```python
from build123d import *

# Parameters (mm, degrees)
SKETCH2_R           = 1.5
BOSS_EXTRUDE1_DEPTH = 2
SKETCH2_4_R         = 4
SKETCH2_4_R_2       = 1.5
BOSS_EXTRUDE2_DEPTH = 20
CUT_EXTRUDE1_START  = 20
SKETCH2_5_R         = 4
SKETCH2_5_R_2       = 3
CUT_EXTRUDE1_DEPTH  = 5


with BuildPart() as part:
    # Sketch2 → Boss-Extrude1 (new body)
    with BuildSketch(Plane(origin=(0, 0, 0), x_dir=(1, 0, 0), z_dir=(0, 1, 0))):
        with BuildLine():
            ThreePointArc((22, -5.5), (27.5, 0), (22, 5.5))
            ThreePointArc((22, 5.5), (16.628166969, 6.705737819), (12.286949473, 10.091623885))
            ThreePointArc((12.286949473, 10.091623885), (11.242997821, 11.242997821), (10.091623885, 12.286949473))
            ThreePointArc((10.091623885, 12.286949473), (6.705737819, 16.628166969), (5.5, 22))
            ThreePointArc((5.5, 22), (0, 27.5), (-5.5, 22))
            ThreePointArc((-5.5, 22), (-6.705737819, 16.628166969), (-10.091623885, 12.286949473))
            ThreePointArc((-10.091623885, 12.286949473), (-11.242997821, 11.242997821), (-12.286949473, 10.091623885))
            ThreePointArc((-12.286949473, 10.091623885), (-16.628166969, 6.705737819), (-22, 5.5))
            ThreePointArc((-22, 5.5), (-27.5, 0), (-22, -5.5))
            ThreePointArc((-22, -5.5), (-16.628166969, -6.705737819), (-12.286949473, -10.091623885))
            ThreePointArc((-12.286949473, -10.091623885), (-11.242997821, -11.242997821), (-10.091623885, -12.286949473))
            ThreePointArc((-10.091623885, -12.286949473), (-6.705737819, -16.628166969), (-5.5, -22))
            ThreePointArc((-5.5, -22), (0, -27.5), (5.5, -22))
            ThreePointArc((5.5, -22), (6.705737819, -16.628166969), (10.091623885, -12.286949473))
            ThreePointArc((10.091623885, -12.286949473), (11.242997821, -11.242997821), (12.286949473, -10.091623885))
            ThreePointArc((12.286949473, -10.091623885), (16.628166969, -6.705737819), (22, -5.5))
        make_face()
        with Locations(Location((-22, 0, 0), (0, 0, 270))):
            Circle(SKETCH2_R, mode=Mode.SUBTRACT)
        with Locations(Location((-9.192388155, -9.192388155, 0), (0, 0, 270))):
            Circle(SKETCH2_R, mode=Mode.SUBTRACT)
        with BuildLine():
            Line((7.526291329, 6.431558041), (7.526291329, 0))
            Line((7.526291329, 0), (7.526291329, -6.388653952))
            Line((7.526291329, -6.388653952), (7.562744256, -6.388653952))
            ThreePointArc((7.562744256, -6.388653952), (-1e-09, -9.9), (-7.562744258, -6.38865395))
            Line((-7.562744258, -6.38865395), (-7.526291329, -6.388653952))
            Line((-7.526291329, -6.388653952), (-7.526291329, 6.431558041))
            ThreePointArc((-7.526291329, 6.431558041), (0, 9.9), (7.526291329, 6.431558041))
        make_face(mode=Mode.SUBTRACT)
        with Locations(Location((0, -22, 0), (0, 0, 270))):
            Circle(SKETCH2_R, mode=Mode.SUBTRACT)
        with Locations(Location((9.192388155, -9.192388155, 0), (0, 0, 270))):
            Circle(SKETCH2_R, mode=Mode.SUBTRACT)
        with Locations(Location((22, 0, 0), (0, 0, 270))):
            Circle(SKETCH2_R, mode=Mode.SUBTRACT)
        with Locations(Location((-9.192388155, 9.192388155, 0), (0, 0, 270))):
            Circle(SKETCH2_R, mode=Mode.SUBTRACT)
        with Locations(Location((9.192388155, 9.192388155, 0), (0, 0, 270))):
            Circle(SKETCH2_R, mode=Mode.SUBTRACT)
        with Locations(Location((0, 22, 0), (0, 0, 270))):
            Circle(SKETCH2_R, mode=Mode.SUBTRACT)
    extrude(amount=BOSS_EXTRUDE1_DEPTH)

    # Sketch2<4> → Boss-Extrude2 (add)
    with BuildSketch(Plane(origin=(0, 0, 0), x_dir=(1, 0, 0), z_dir=(0, 1, 0))):
        with Locations(Location((22, 0, 0), (0, 0, 270))):
            Circle(SKETCH2_4_R)
        with Locations(Location((22, 0, 0), (0, 0, 270))):
            Circle(SKETCH2_4_R_2, mode=Mode.SUBTRACT)
        with Locations(Location((0, -22, 0), (0, 0, 270))):
            Circle(SKETCH2_4_R)
        with Locations(Location((0, -22, 0), (0, 0, 270))):
            Circle(SKETCH2_4_R_2, mode=Mode.SUBTRACT)
        with Locations(Location((-22, 0, 0), (0, 0, 270))):
            Circle(SKETCH2_4_R)
        with Locations(Location((-22, 0, 0), (0, 0, 270))):
            Circle(SKETCH2_4_R_2, mode=Mode.SUBTRACT)
        with Locations(Location((0, 22, 0), (0, 0, 270))):
            Circle(SKETCH2_4_R)
        with Locations(Location((0, 22, 0), (0, 0, 270))):
            Circle(SKETCH2_4_R_2, mode=Mode.SUBTRACT)
    extrude(amount=BOSS_EXTRUDE2_DEPTH)

    # Sketch2<5> → Cut-Extrude1 (cut)
    with BuildSketch(Plane(origin=(0, 0, 0), x_dir=(1, 0, 0), z_dir=(0, 1, 0)).offset(CUT_EXTRUDE1_START)):
        with Locations(Location((-22, 0, 0), (0, 0, 270))):
            Circle(SKETCH2_5_R)
        with Locations(Location((-22, 0, 0), (0, 0, 270))):
            Circle(SKETCH2_5_R_2, mode=Mode.SUBTRACT)
        with Locations(Location((0, 22, 0), (0, 0, 270))):
            Circle(SKETCH2_5_R)
        with Locations(Location((0, 22, 0), (0, 0, 270))):
            Circle(SKETCH2_5_R_2, mode=Mode.SUBTRACT)
        with BuildLine():
            ThreePointArc((19, 0), (22, 3), (25, 0))
            Line((25, 0), (26, 0))
            ThreePointArc((26, 0), (22, 4), (18, 0))
            Line((18, 0), (19, 0))
        make_face()
        with BuildLine():
            Line((26, 0), (25, 0))
            ThreePointArc((25, 0), (22, -3), (19, 0))
            Line((19, 0), (18, 0))
            ThreePointArc((18, 0), (22, -4), (26, 0))
        make_face()
        with Locations(Location((0, -22, 0), (0, 0, 270))):
            Circle(SKETCH2_5_R)
        with Locations(Location((0, -22, 0), (0, 0, 270))):
            Circle(SKETCH2_5_R_2, mode=Mode.SUBTRACT)
    extrude(amount=-CUT_EXTRUDE1_DEPTH, mode=Mode.SUBTRACT)


solid = part.part
```
Geometry: final body of the model. Coordinates: model frame, mm. A direction names the side the tool comes from. Round coordinates to 2 decimals unless told otherwise and drop trailing zeros. Loops run counter-clockwise (first coordinate to the right, second up) from the corner with the lowest first, then second, coordinate; pieces in that order, holes last. Notation, with made-up numbers: (24, 14.5) -> (52, 14.5) arc R14 cw to (52, 23.5) -> close; hole circle Ø7 at (-9, 61). An arc over 180 degrees is marked (long way). Use one line per item in the form item = value.
Item 1: Cut plane B-B on x = 0. Give the number of separate pieces and of enclosed holes in the cut face, then the cut area to 3 significant figures.
Evaluation:
separate_pieces = 4
enclosed_holes = 0
area = 218 mm2
Item 2: Draft query along Z for faces 4 (the cylindrical face through (16.7, 0.99, -6.67)), 5 (the cylindrical face through (16.56, 0.99, 6.74)), 6 (the cylindrical face through (-18.034, 8.409, -0.521)), 7 (the cylindrical face through (7.86, 0.99, 9.88)). Return one class per face: released by +Z, released by -Z, zero draft, split by the parting line, or undercut.
Evaluation:
face_4 = released by -Z
face_5 = released by +Z
face_6 = split by the parting line
face_7 = undercut
Item 3: Access query for faces 1 (the flat face through (-23.3, 20, 1.3)), 2 (the cylindrical face through (19, 18, 0)), 3 (the flat face through (7.526, 1, 0)). Directions: +Z, -Z, +X, -X, +Y, -Y. A direction counts if a zero-diameter tool reaches every point of the face in a straight line with its end or side. Return the directions, or none.
Evaluation:
face_1 = +Z, -Z, +X, -X, +Y
face_2 = +Y
face_3 = +Y, -Y
Item 4: Cut plane D-D on y = 15.75. Output: boundary loops of the cut face in (x, z), then the cut area to 3 significant figures.
Evaluation:
outline = circle Ø6 at (-22, 0); circle Ø6 at (0, -22); circle Ø6 at (0, 22); circle Ø6 at (22, 0); hole circle Ø3 at (-22, 0); hole circle Ø3 at (0, -22); hole circle Ø3 at (0, 22); hole circle Ø3 at (22, 0)
area = 84.8 mm2
Item 5: Contact query for flat-ended pins moving along their axis: pin 1 Ø6 at (y, z) = (2, 10.5) entering from +X; pin 2 Ø10 at (y, z) = (4, -18.5) entering from -X; pin 3 Ø1.6 at (y, z) = (1, 1.5) entering from -X; pin 4 Ø5 at (x, z) = (-22, 0) entering from +Y. Output: stop coordinate, or through.
Evaluation:
pin_1 = 15.2
pin_2 = -8.44
pin_3 = -27.46
pin_4 = 20
Item 6: Cut plane A-A on y = 8. Output: boundary loops of the cut face in (x, z), then the cut area to 3 significant figures.
Evaluation:
outline = circle Ø8 at (-22, 0); circle Ø8 at (0, -22); circle Ø8 at (0, 22); circle Ø8 at (22, 0); hole circle Ø3 at (-22, 0); hole circle Ø3 at (0, -22); hole circle Ø3 at (0, 22); hole circle Ø3 at (22, 0)
area = 173 mm2
Item 7: Material intervals for probe 1 along X at (y, z) = (7, 0); probe 2 along X at (y, z) = (7, 1); probe 3 along Z at (x, y) = (-0.5, 1.25), sorted ascending.
Evaluation:
probe_1 = -26 to -23.5, -20.5 to -18, 18 to 20.5, 23.5 to 26
probe_2 = -25.87 to -23.12, -20.88 to -18.13, 18.13 to 20.88, 23.12 to 25.87
probe_3 = -27.48 to -23.41, -20.59 to -9.89, 9.89 to 20.59, 23.41 to 27.48
